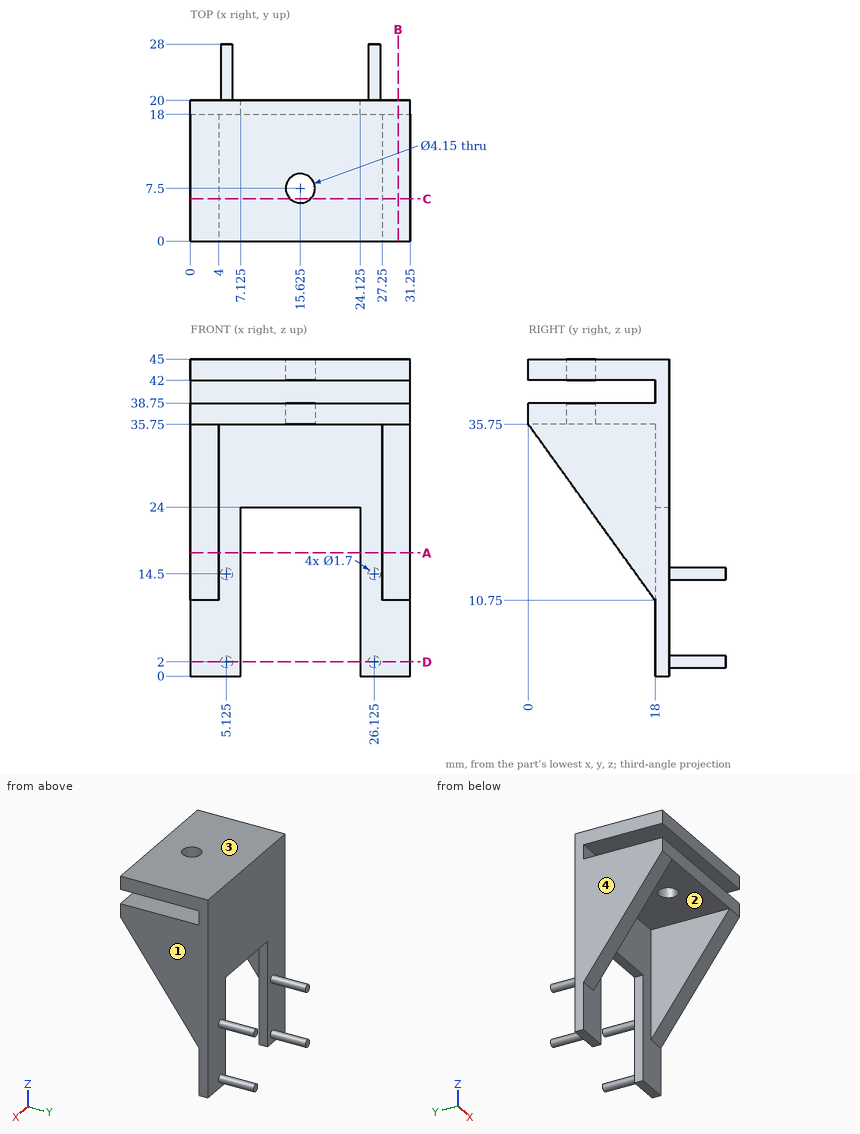
Answer from the drawing. Dimensions are ordinates in mm from the lowest x, y and z of the part. Coordinates: 2 decimals unless noted, no trailing zeros. Order: outer loops, then holes, each group sorted by start corner. A loop starts at its lowest first (then second) coordinate and runs counter-clockwise, first axis right, second up. Notation, with made-up numbers: M 78.25,54 L 85.25,54 A9 cw 85.25,69 Z; hole C 45,-4 d9. An arc over 180 degrees is marked long. Put each result on its own line as item: value. Start each with the question number.
Item 1: Section A-A, the plane z = 17.5 is taken. Determine the outline of the cut face in (x, y) (3 decimals).
Item 2: Section B-B, the plane x = 29.5 is taken. Determine the outline of the cut face in (y, z).
Item 3: The mould has two halves that part along X. Classify the marked faces 1, 2, 3 and 4: +X half, -X half, draft (parallel to the pull), parting line (faces both ways), or undercut.
Item 4: Section C-C, the plane y = 6 is taken. Determine the outline of the cut face in (x, z).
Item 5: Given pin 1 Ø8 at (x, z) = (23.5, 7) entering from -Y; pin 2 Ø14.5 at (x, y) = (19.5, 11.5) entering from -Z; pin 3 Ø3.5 at (x, y) = (15.625, 7.5) entering from +Z, each flat-ended and moving along its own axis, determine where each tip first touches the part or whether it passes through.
Item 6: Consider probe 1 along Z at (x, y) = (5, 11.5); probe 2 along X at (y, z) = (12, 31). Determine where each line is inside the solid, lowest interval first. Write a range as [from, to].
Item 7: Section D-D, the plane z = 2 is taken. Determine the outline of the cut face in (x, y) (3 decimals).
Computed:
1. outline: M 0,13.14 L 4,13.14 L 4,18 L 7.125,18 L 7.125,20 L 0,20 Z; M 24.125,18 L 27.25,18 L 27.25,13.14 L 31.25,13.14 L 31.25,20 L 24.125,20 Z
2. outline: M 0,35.75 L 18,10.75 L 18,0 L 20,0 L 20,45 L 0,45 L 0,42 L 18,42 L 18,38.75 L 0,38.75 Z
3. face 1: +X half
3. face 2: undercut
3. face 3: draft
3. face 4: -X half
4. outline: M 0,27.42 L 4,27.42 L 4,35.75 L 14.19,35.75 L 14.19,38.75 L 0,38.75 Z; M 0,42 L 14.19,42 L 14.19,45 L 0,45 Z; M 17.06,35.75 L 27.25,35.75 L 27.25,27.42 L 31.25,27.42 L 31.25,38.75 L 17.06,38.75 Z; M 17.06,42 L 31.25,42 L 31.25,45 L 17.06,45 Z
5. pin 1: stops at y = 18
5. pin 2: stops at z = 24
5. pin 3: passes through
6. probe 1: z = [35.75, 38.75], [42, 45]
6. probe 2: x = [0, 4], [27.25, 31.25]
7. outline: M 0,18 L 7.125,18 L 7.125,20 L 5.975,20 L 5.975,28 L 4.275,28 L 4.275,20 L 0,20 Z; M 24.125,18 L 31.25,18 L 31.25,20 L 26.975,20 L 26.975,28 L 25.275,28 L 25.275,20 L 24.125,20 Z
